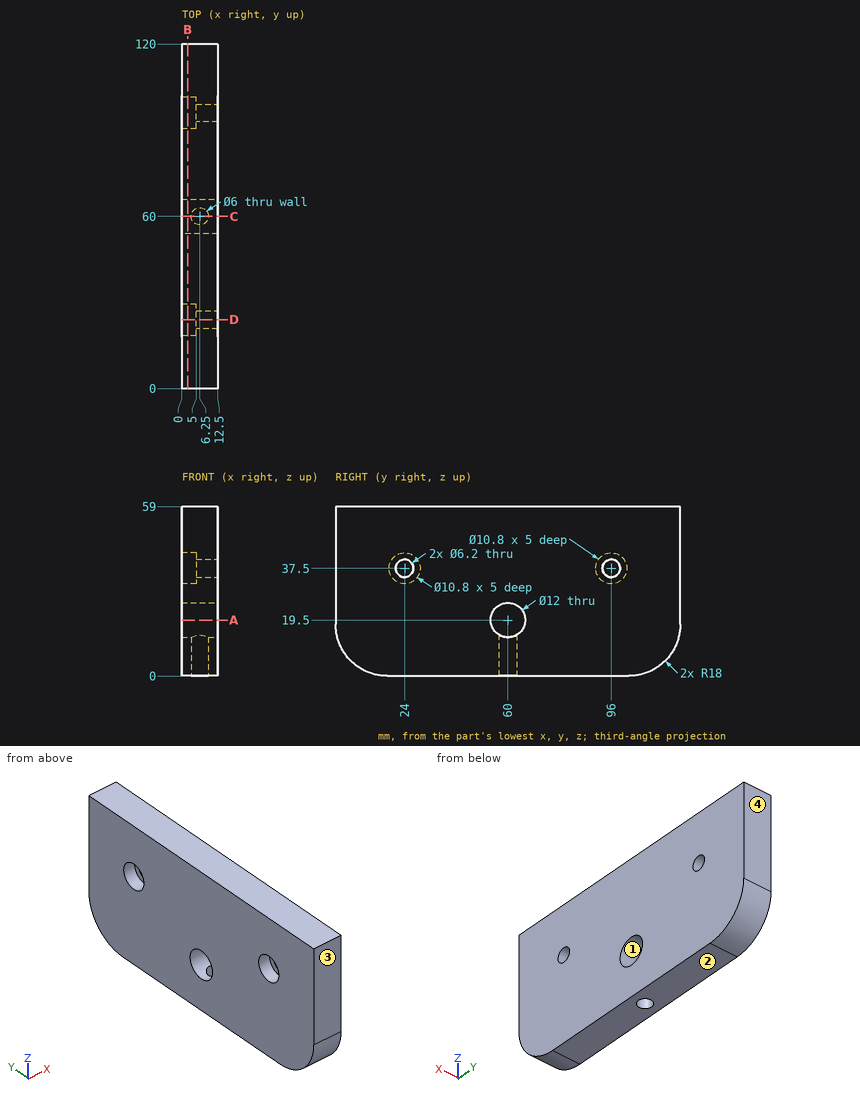
Check sheet for the drawn part. Datum: minimum x, y, z corner. Units: mm. Coordinates: 2 decimals unless noted, no trailing zeros. Order: outer loops, then holes, each group sorted by start corner. A loop starts at its lowest first (then second) coordinate and runs counter-clockwise, first axis right, second up. Notation, with made-up numbers: (-18.75, 46) -> (33.25, 46) arc R26 cw to (33.25, 62) -> close; hole circle Ø10 at (63.5, 23.5). An arc over 180 degrees is marked (long way). Use a Markdown table: item, result. Add a question column.
1. Go/stop test with flat-tipped pins: pin 1 Ø5.5 at (y, z) = (96, 37.5) entering from -X; pin 2 Ø8.5 at (y, z) = (24, 37.5) entering from -X; pin 3 Ø4 at (x, z) = (8.5, 35.5) entering from -Y; pin 4 Ø1.5 at (x, z) = (10.5, 13.5) entering from +Y. Record where each tip stops, or that it passes through.
2. Cross-section at C-C (y = 60). Enter the section's corners in (x, z), and give its area (4 significant figures).
3. Cross-section at B-B (x = 2). Enter the section's corners in (y, z).
4. Cross-section at A-A (z = 19.5). Enter the section's corners in (x, y), and give its area (3 significant figures).
5. Material ranges on L1, parallel to X at y = 60, z = 7; L2, parallel to Z at x = 2.7, y = 24; L3, parallel to Z at x = 6.75, y = 24, recorded low to high.
6. Cross-section at D-D (y = 24). Enter the section's corners in (x, z), and give its area (3 significant figures).
7. Mould release check, pull along Y, two halves, no side actions. Record for the marked faces 1, 2, 3 and 4: pulls with the +Y half, pulls with the -Y half, needs draft (parallel to the pull), parting line crosses it, or undercut.
Filled sheet:
| question | item | result |
|---|---|---|
| 1 | pin 1 | through |
| 1 | pin 2 | x = 5 |
| 1 | pin 3 | y = 0 |
| 1 | pin 4 | y = 119.61 |
| 2 | outline | (0, 0) -> (3.25, 0) -> (3.25, 13.5) -> (0, 13.5) -> close; (0, 25.5) -> (12.5, 25.5) -> (12.5, 59) -> (0, 59) -> close; (9.25, 0) -> (12.5, 0) -> (12.5, 13.5) -> (9.25, 13.5) -> close |
| 2 | area | 506.5 mm2 |
| 3 | outline | (0, 18) arc R18 ccw to (18, 0) -> (102, 0) arc R18 ccw to (120, 18) -> (120, 59) -> (0, 59) -> close; hole circle Ø10.8 at (24, 37.5); hole circle Ø12 at (60, 19.5); hole circle Ø10.8 at (96, 37.5) |
| 4 | outline | (0, 0) -> (12.5, 0) -> (12.5, 54) -> (0, 54) -> close; (0, 66) -> (12.5, 66) -> (12.5, 120) -> (0, 120) -> close |
| 4 | area | 1,350 mm2 |
| 5 | L1 | 0 to 3.25, 9.25 to 12.5 |
| 5 | L2 | 0 to 32.1, 42.9 to 59 |
| 5 | L3 | 0 to 34.4, 40.6 to 59 |
| 6 | outline | (0, 0) -> (12.5, 0) -> (12.5, 34.4) -> (5, 34.4) -> (5, 32.1) -> (0, 32.1) -> close; (0, 42.9) -> (5, 42.9) -> (5, 40.6) -> (12.5, 40.6) -> (12.5, 59) -> (0, 59) -> close |
| 6 | area | 637 mm2 |
| 7 | face 1 | undercut |
| 7 | face 2 | needs draft |
| 7 | face 3 | pulls with the -Y half |
| 7 | face 4 | pulls with the +Y half |
